from build123d import *

# Parameters (mm, degrees)
SKETCH1_R           = 3.5
SKETCH1_R_2         = 1.5
SKETCH1_W           = 15.74389133
SKETCH1_H           = 26.239818884
BOSS_EXTRUDE1_DEPTH = 3
FILLET1_R           = 3
SKETCH2_W           = 11.534893024
SKETCH2_H           = 5.633319849
BOSS_EXTRUDE2_DEPTH = 5


with BuildPart() as part:
    # Sketch1 → Boss-Extrude1 (new body)
    # profile 1 of 5: a face of its own
    with BuildSketch(Plane(origin=(0, 0, 0), x_dir=(1, 0, 0), z_dir=(0, 1, 0))):
        with Locations((9, 15)):
            Circle(SKETCH1_R)
        with Locations(Location((9, 15, 0), (0, 0, 270))):
            Circle(SKETCH1_R_2, mode=Mode.SUBTRACT)
    # profile 2 of 5: a face of its own
    with BuildSketch(Plane(origin=(0, 0, 0), x_dir=(1, 0, 0), z_dir=(0, 1, 0))):
        with Locations((9, -15)):
            Circle(SKETCH1_R)
        with Locations(Location((9, -15, 0), (0, 0, 270))):
            Circle(SKETCH1_R_2, mode=Mode.SUBTRACT)
    # profile 3 of 5: a face of its own
    with BuildSketch(Plane(origin=(0, 0, 0), x_dir=(1, 0, 0), z_dir=(0, 1, 0))):
        with Locations((-9, -15)):
            Circle(SKETCH1_R)
        with Locations(Location((-9, -15, 0), (0, 0, 270))):
            Circle(SKETCH1_R_2, mode=Mode.SUBTRACT)
    # profile 4 of 5: a face of its own
    with BuildSketch(Plane(origin=(0, 0, 0), x_dir=(1, 0, 0), z_dir=(0, 1, 0))):
        with Locations((-9, 15)):
            Circle(SKETCH1_R)
        with Locations(Location((-9, 15, 0), (0, 0, 270))):
            Circle(SKETCH1_R_2, mode=Mode.SUBTRACT)
    # profile 5 of 5: a face of its own
    with BuildSketch(Plane(origin=(0, 0, 0), x_dir=(1, 0, 0), z_dir=(0, 1, 0))):
        Rectangle(SKETCH1_W, SKETCH1_H)
    extrude(amount=BOSS_EXTRUDE1_DEPTH)

    # Fillet1
    fillet1_edges = [part.edges().sort_by_distance(p)[0] for p in [
        (-6.047838166, 1.5, -13.119909442),
        (6.047838166, 1.5, -13.119909442),
        (7.871945665, 1.5, -11.686769942),
        (7.871945665, 1.5, 11.686769942),
        (6.047838166, 1.5, 13.119909442),
        (-6.047838166, 1.5, 13.119909442),
        (-7.871945665, 1.5, 11.686769942),
        (-7.871945665, 1.5, -11.686769942),
    ]]
    fillet(fillet1_edges, radius=FILLET1_R)

    # Sketch2 → Boss-Extrude2 (add)
    with BuildSketch(Plane(origin=(0, 3, 0), x_dir=(1, 0, 0), z_dir=(0, 1, 0))):
        with Locations((0, 9.898547735)):
            Rectangle(SKETCH2_W, SKETCH2_H)
        with Locations((0, -9.898547735)):
            Rectangle(SKETCH2_W, SKETCH2_H)
    extrude(amount=BOSS_EXTRUDE2_DEPTH)


solid = part.part
Input: part model. Units: mm. Frame: model coordinates. A direction names the side the tool comes from. Coordinates: 2 decimals unless noted, no trailing zeros. Loops run counter-clockwise (first coordinate to the right, second up) from the corner with the lowest first, then second, coordinate; pieces in that order, holes last.
Q1. Draft query along X for faces 5 (the face through (0, 5, 7.082)), 6 (the face through (11.4, 1.48, -17.55)), 7 (the face through (-8.449, 1.479, 10.544)), 8 (the face through (7.872, 1, 0)). Return one class per face: +X half, -X half, draft (parallel to the pull), parting line (faces both ways), or undercut.
Q2. Material intervals for line 1 (Z direction, x = 4, y = 5.5); line 2 (X direction, y = 1.55, z = -15); line 3 (Z direction, x = -8.5, y = 1.5), sorted ascending.
Q3. Contact query for flat-ended pins moving along their axis: pin 1 (0.9 mm diameter, centred on x = 1, y = 1.5, fed in from +Z); pin 2 (3.5 mm diameter, centred on x = -9, z = 15, fed in from -Y); pin 3 (2 mm diameter, centred on y = 5.5, z = -4, fed in from -X); pin 4 (2.5 mm diameter, centred on y = 1.5, z = 1.5, fed in from -X). Output: stop coordinate, or through.
Q4. Cut plane B-B (z = 15). Output: boundary loops of the cut face in (x, y).
Q5. Cut plane A-A (y = 4.25). Output: boundary loops of the cut face in (x, z), then the cut area to 3 significant figures.
Q6. Set-up query: faces 1 (the face through (0, 5, -7.082)), 2 (the face through (-5.767, 5, -10)), 3 (the face through (0, 1, -13.12)), 4 (the face through (4.5, 1.5, 13.8)). Return all of +Z, -Z, +X, -X, +Y, -Y with unobstructed straight access to the full face (end or side cutting, diameter ignored); none if empty.
Q7. Cut plane C-C (x = -9). Output: boundary loops of the cut face in (y, z), then the cut area to 3 significant figures.
Q8. Cut plane D-D (z = -4). Output: boundary loops of the cut face in (x, y), then the cut area to 3 significant figures.
Working result:
1. face 5: draft
1. face 6: undercut
1. face 7: -X half
1. face 8: +X half
2. line 1: z = -12.72 to -7.08, 7.08 to 12.72
2. line 2: x = -12.5 to -10.5, -7.5 to -5.38, 5.38 to 7.5, 10.5 to 12.5
2. line 3: z = -18.46 to -16.41, -13.59 to -10.61, 10.61 to 13.59, 16.41 to 18.46
3. pin 1: stops at z = 13.12
3. pin 2: stops at y = 0
3. pin 3: passes through
3. pin 4: stops at x = -7.87
4. outline: (-12.5, 0) - (-10.5, 0) - (-10.5, 3) - (-12.5, 3) - close; (-7.5, 0) - (-5.38, 0) - (-5.38, 3) - (-7.5, 3) - close; (5.38, 0) - (7.5, 0) - (7.5, 3) - (5.38, 3) - close; (10.5, 0) - (12.5, 0) - (12.5, 3) - (10.5, 3) - close
5. outline: (-5.77, -12.72) - (5.77, -12.72) - (5.77, -7.08) - (-5.77, -7.08) - close; (-5.77, 7.08) - (5.77, 7.08) - (5.77, 12.72) - (-5.77, 12.72) - close
5. area: 130 mm2
6. face 1: +X, -X, +Y
6. face 2: +Z, -Z, -X, +Y
6. face 3: -Z, +Y, -Y
6. face 4: +Z, +Y, -Y
7. outline: (0, -18.5) - (3, -18.5) - (3, -16.5) - (0, -16.5) - close; (0, -13.5) - (3, -13.5) - (3, -11.12) - (0, -11.12) - close; (0, 11.12) - (3, 11.12) - (3, 13.5) - (0, 13.5) - close; (0, 16.5) - (3, 16.5) - (3, 18.5) - (0, 18.5) - close
7. area: 26.3 mm2
8. outline: (-7.87, 0) - (7.87, 0) - (7.87, 3) - (-7.87, 3) - close
8. area: 47.2 mm2
